from build123d import *

# Parameters (mm, degrees)
F1_DEPTH = 2
F2_W     = 7
F2_H     = 6
F3_DEPTH = 2
F5_DEPTH = 6.5
F7_DEPTH = 6.5


with BuildPart() as f1:
    # F0 (on Top) → F1 (new body)
    with BuildSketch(Plane.XY):
        with BuildLine():
            Line((-40, -16), (-40, 0))
            Line((-40, 0), (-58, 0))
            Line((-58, 0), (-58, -14.978968))
            ThreePointArc((-58, -14.978968), (-57.12132, -17.100288), (-55, -17.978968))
            Line((-55, -17.978968), (-40.289286, -17.978968))
            ThreePointArc((-40.289286, -17.978968), (-30.191853, -20.92634), (-21.289286, -26.528968))
            Line((-21.289286, -26.528968), (-18.710714, -26.528968))
            ThreePointArc((-18.710714, -26.528968), (-9.808147, -20.92634), (0.289286, -17.978968))
            Line((0.289286, -17.978968), (15, -17.978968))
            ThreePointArc((15, -17.978968), (17.12132, -17.100288), (18, -14.978968))
            Line((18, -14.978968), (18, 0))
            Line((18, 0), (0, 0))
            Line((0, 0), (0, -16))
            ThreePointArc((0, -16), (-10.628876, -19.102497), (-20, -25))
            ThreePointArc((-20, -25), (-29.371124, -19.102497), (-40, -16))
        make_face()
    extrude(amount=F1_DEPTH)

    # F2 (on face) → F3 (cut, through all)
    with BuildSketch(Plane.XY.offset(2)):
        with Locations((-48, -3)):
            Rectangle(F2_W, F2_H)
        with Locations((8, -3)):
            Rectangle(F2_W, F2_H)
    extrude(amount=-F3_DEPTH, mode=Mode.SUBTRACT)

    # F4 (on face) → F5 (join, through all)
    with BuildSketch(Plane(origin=(-58, 0, 0), x_dir=(0, -1, 0), z_dir=(-1, 0, 0))):
        Polygon((4.5, 4.3), (3, 2), (5, 2), (5, 4.3), align=None)
    extrude(amount=-F5_DEPTH)

    # F6 (on face) → F7 (join, through all)
    with BuildSketch(Plane.YZ.offset(18)):
        Polygon((-3, 2), (-4.5, 4.3), (-5, 4.3), (-5, 2), align=None)
    extrude(amount=-F7_DEPTH)


solid = f1.part
Model file for the job. Use its own axes, mm. A direction names the side the tool comes from. Coordinates: 2 decimals unless noted, no trailing zeros. Write each loop counter-clockwise with the first axis right and the second up, starting at its lowest first coordinate (ties: lowest second). Pieces come first, ordered by that corner, then holes. Notation, with made-up numbers: (-9.5, 18) - (11.5, 18) arc R21 cw to (11.5, 54) - close; hole circle Ø10 at (72, 2.5). An arc over 180 degrees is marked (long way). Write each question's results on one line, items separated by ' | '. Start each with the question number.
1) Mould opens along X. For faces 5 (the face through (18, -8, 1)), 6 (the face through (8, -17.979, 1)), 7 (the face through (-10.49, -19.04, 0.99)), 8 (the face through (-30.327, -20.866, 0.986)) say: pulls with the +X half, pulls with the -X half, needs draft (parallel to the pull), parting line crosses it, or undercut.
2) Cut at C-C (x = 12.5). Write the cut outline in (y, z), then the cut area to 3 significant figures.
3) Flat gauge pins, fed straight in: P1, Ø0.6, axis at x = -49.5, z = 0.5, coming from the +Y side; P2, Ø1, axis at x = -51, z = 1, coming from the -Y side; P3, Ø10, axis at x = 6.5, y = -18.5, coming from the +Z side; P4, Ø2, axis at y = -3, z = 3, coming from the +X side. Where does each tip first touch, or does it go through?
4) Cut at B-B (y = -12.5). Write the cut outline in (x, z), then the cut area to 3 significant figures.
5) Probe line 1 along X through (y, z) = (-8.25, 1.8); line 2 along Y through (x, z) = (8, 0.6); line 3 along Z through (x, y) = (-31.5, -19.25). List the from-to ranges inside material, lowest first. Write a range as from..to.
6) Cut at D-D (z = 3.6). Write the cut outline in (x, y), then the cut area to 3 significant figures.
7) 3-axis set-ups, long thin cutter, end or side, ignore diameter. For faces 1 (the face through (-48, -17.979, 1)), 2 (the face through (4.5, -3, 1)), 3 (the face through (14.796, -3.74, 3.134)), 4 (the face through (-55, -5, 3)): which of +Z, -Z, +X, -X, +Y, -Y reach the whole face in a straight line?
8) Cut at A-A (y = -2). Write the cut outline in (x, z), then the cut area to 3 significant figures.
Returned:
1) face 5: pulls with the +X half | face 6: needs draft | face 7: undercut | face 8: pulls with the -X half
2) outline: (-17.98, 0) - (0, 0) - (0, 2) - (-3, 2) - (-4.5, 4.3) - (-5, 4.3) - (-5, 2) - (-17.98, 2) - close | area: 38.8 mm^2
3) P1: y = -6 | P2: y = -17.98 | P3: z = 2 | P4: x = 18
4) outline: (-58, 0) - (-40, 0) - (-40, 2) - (-58, 2) - close; (0, 0) - (18, 0) - (18, 2) - (0, 2) - close | area: 72.0 mm^2
5) line 1: -58..-40, 0..18 | line 2: -17.98..-6 | line 3: 0..2
6) outline: (-58, -5) - (-51.5, -5) - (-51.5, -4.04) - (-58, -4.04) - close; (11.5, -5) - (18, -5) - (18, -4.04) - (11.5, -4.04) - close | area: 12.4 mm^2
7) face 1: +Z, -Z, -X, -Y | face 2: +Z, -Z, +Y | face 3: +Z, +X, -X, +Y | face 4: +Z, +X, -X, -Y
8) outline: (-58, 0) - (-51.5, 0) - (-51.5, 2) - (-58, 2) - close; (-44.5, 0) - (-40, 0) - (-40, 2) - (-44.5, 2) - close; (0, 0) - (4.5, 0) - (4.5, 2) - (0, 2) - close; (11.5, 0) - (18, 0) - (18, 2) - (11.5, 2) - close | area: 44.0 mm^2
